Can you work these out from the model? Positions are in its coordinate system, mm. Face numbers are marked on the shaded views. A direction names the side the tool comes from. Coordinates: 2 decimals unless noted, no trailing zeros. Order: outer loops, then holes, each group sorted by start corner. A loop starts at its lowest first (then second) coordinate and runs counter-clockwise, first axis right, second up. Notation, with made-up numbers: (-29, -25.5) -> (-10, -25.5) arc R9 ccw to (-10, -13.5) -> close; hole circle Ø4 at (1, 87). An arc over 180 degrees is marked (long way). Write item = value, one per line.
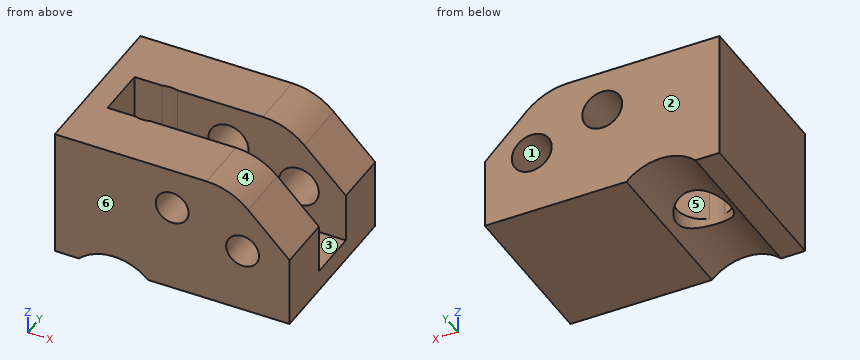
```python
from build123d import *

# Parameters (mm, degrees)
CYLINDER060_R          = 2.3
CYLINDER060_DEPTH      = 62
CYLINDER062_R          = 4.2
CYLINDER062_DEPTH      = 24
CYLINDER062_ROLL_ANGLE = 90
BOX001024_W            = 23
BOX001024_H            = 4.4
BOX001024_DEPTH        = 13
CYLINDER056_R          = 1.7
CYLINDER056_DEPTH      = 20
CYLINDER056_ROLL_ANGLE = 90
CYLINDER057_R          = 1.7
CYLINDER057_DEPTH      = 20
CYLINDER057_ROLL_ANGLE = 90
CYLINDER059_R          = 1.4
CYLINDER059_DEPTH      = 20
CYLINDER059_ROLL_ANGLE = 90
CYLINDER058_R          = 1.4
CYLINDER058_DEPTH      = 20
CYLINDER058_ROLL_ANGLE = 90
BOX001025_W            = 10
BOX001025_H            = 27
BOX001025_DEPTH        = 10
BOX001022_W            = 23
BOX001022_H            = 14
BOX001022_DEPTH        = 11
CHAMFER003_SIZE        = 8
FILLET007_R            = 5


with BuildPart() as cylinder060:
    # Cylinder060 → Cylinder060 (new body)
    with BuildSketch(Plane.XY.offset(-56)):
        Circle(CYLINDER060_R)
    extrude(amount=CYLINDER060_DEPTH)


with BuildPart() as cylinder062:
    # Cylinder062 → Cylinder062 (new body)
    with BuildSketch(Plane.XY):
        Circle(CYLINDER062_R)
    extrude(amount=CYLINDER062_DEPTH)


with BuildPart() as cylinder062_1:
    # Cylinder062 roll: moved
    add(cylinder062.part.rotate(Axis((0, 0, 0), (1, 0, 0)), CYLINDER062_ROLL_ANGLE))


with BuildPart() as cylinder062_2:
    # Cylinder062 placement: moved
    add(cylinder062_1.part.moved(Location((0, 11, -52))))


with BuildPart() as cube022:
    # Box001024 → Box001024 (new body)
    with BuildSketch(Plane(origin=(-3, -2.2, -47.2), x_dir=(1, 0, 0), z_dir=(0, 0, 1))):
        with Locations((11.5, 2.2)):
            Rectangle(BOX001024_W, BOX001024_H)
    extrude(amount=BOX001024_DEPTH)


with BuildPart() as cylinder056:
    # Cylinder056 → Cylinder056 (new body)
    with BuildSketch(Plane.XY):
        Circle(CYLINDER056_R)
    extrude(amount=CYLINDER056_DEPTH)


with BuildPart() as cylinder056_1:
    # Cylinder056 roll: moved
    add(cylinder056.part.rotate(Axis((0, 0, 0), (1, 0, 0)), CYLINDER056_ROLL_ANGLE))


with BuildPart() as cylinder056_2:
    # Cylinder056 placement: moved
    add(cylinder056_1.part.moved(Location((11, 19, -43.5))))


with BuildPart() as cylinder057:
    # Cylinder057 → Cylinder057 (new body)
    with BuildSketch(Plane.XY):
        Circle(CYLINDER057_R)
    extrude(amount=CYLINDER057_DEPTH)


with BuildPart() as cylinder057_1:
    # Cylinder057 roll: moved
    add(cylinder057.part.rotate(Axis((0, 0, 0), (1, 0, 0)), CYLINDER057_ROLL_ANGLE))


with BuildPart() as cylinder057_2:
    # Cylinder057 placement: moved
    add(cylinder057_1.part.moved(Location((5, 19, -41.5))))


with BuildPart() as cylinder059:
    # Cylinder059 → Cylinder059 (new body)
    with BuildSketch(Plane.XY):
        Circle(CYLINDER059_R)
    extrude(amount=CYLINDER059_DEPTH)


with BuildPart() as cylinder059_1:
    # Cylinder059 roll: moved
    add(cylinder059.part.rotate(Axis((0, 0, 0), (1, 0, 0)), CYLINDER059_ROLL_ANGLE))


with BuildPart() as cylinder059_2:
    # Cylinder059 placement: moved
    add(cylinder059_1.part.moved(Location((5, -1, -41.5))))


with BuildPart() as fusion074:
    # Cylinder058 → Cylinder058 (new body)
    with BuildSketch(Plane.XY):
        Circle(CYLINDER058_R)
    extrude(amount=CYLINDER058_DEPTH)


with BuildPart() as fusion074_1:
    # Cylinder058 roll: moved
    add(fusion074.part.rotate(Axis((0, 0, 0), (1, 0, 0)), CYLINDER058_ROLL_ANGLE))


with BuildPart() as fusion074_2:
    # Cylinder058 placement: moved
    add(fusion074_1.part.moved(Location((11, -1, -43.5))))

    # Fusion074: union Cylinder056, Cylinder057, Cylinder059
    add(cylinder056_2.part)
    add(cylinder057_2.part)
    add(cylinder059_2.part)


with BuildPart() as cube023:
    # Box001025 → Box001025 (new body)
    with BuildSketch(Plane(origin=(15, -13, -44), x_dir=(1, 0, 0), z_dir=(0, 0, 1))):
        with Locations((5, 13.5)):
            Rectangle(BOX001025_W, BOX001025_H)
    extrude(amount=BOX001025_DEPTH)


with BuildPart() as cut_lever_block:
    # Box001022 → Box001022 (new body)
    with BuildSketch(Plane(origin=(-5, -7, -42), x_dir=(1, 0, 0), z_dir=(0, 0, 1))):
        with Locations((11.5, 7)):
            Rectangle(BOX001022_W, BOX001022_H)
    extrude(amount=BOX001022_DEPTH)

    # Chamfer003
    chamfer003_edges = [cut_lever_block.edges().sort_by_distance(p)[0] for p in [
        (18, 0, -31),
    ]]
    chamfer(chamfer003_edges, length=CHAMFER003_SIZE)

    # Fillet007
    fillet007_edges = [cut_lever_block.edges().sort_by_distance(p)[0] for p in [
        (10, 0, -31),
    ]]
    fillet(fillet007_edges, radius=FILLET007_R)

    # Cut022: cut Cube023
    add(cube023.part, mode=Mode.SUBTRACT)


with BuildPart() as cut_lever_block_1:
    # Cut022 placement: moved
    add(cut_lever_block.part.moved(Location((0, 0, -7))))

    # Cut027: cut Fusion074
    add(fusion074_2.part, mode=Mode.SUBTRACT)

    # Cut028: cut Cube022
    add(cube022.part, mode=Mode.SUBTRACT)

    # Cut029: cut Cylinder062
    add(cylinder062_2.part, mode=Mode.SUBTRACT)

    # Cut030: cut Cylinder060
    add(cylinder060.part, mode=Mode.SUBTRACT)


with BuildPart() as cut_lever_block_2:
    # Cut030 placement: moved
    add(cut_lever_block_1.part.moved(Location((0, 0, -6))))


solid = cut_lever_block_2.part
```
Item 1: I'm going to push flat-ended pins straight in: P1, Ø1.3, axis at x = 11.5, y = 0, coming from the +Z side; P2, Ø2, axis at y = -0.5, z = -46.5, coming from the +X side. Where does each tip first touch, or does it pass through?
A:
P1 = -53.2
P2 = -3
Item 2: I want a section at D-D, the plane x = 5. Please give me the cut outline in (y, z).
A:
outline = (-7, -55) -> (7, -55) -> (7, -49.2) -> (2.2, -49.2) -> (2.2, -53.2) -> (-2.2, -53.2) -> (-2.2, -48.9) -> (-7, -48.9) -> close; (-7, -46.1) -> (-2.2, -46.1) -> (-2.2, -44) -> (-7, -44) -> close; (2.2, -45.8) -> (7, -45.8) -> (7, -44) -> (2.2, -44) -> close
Item 3: If we mould it in two halves opening along Y, with no side actions, what happens to the marked faces 4, 5 and 6? For each: pulls with the +Y half, pulls with the -Y half, needs draft (parallel to the pull), parting line crosses it, or undercut.
A:
face_4 = needs draft
face_5 = undercut
face_6 = pulls with the -Y half
Item 4: I want a section at B-B, the plane z = -49.5. Please give me the cut outline in (x, y), plus the area to 3 significant figures.
A:
outline = (-5, -7) -> (9.6, -7) -> (9.6, -2.2) -> (0.67, -2.2) arc R2.3 cw to (-0.67, -2.2) -> (-3, -2.2) -> (-3, 2.2) -> (-0.67, 2.2) arc R2.3 cw to (0.67, 2.2) -> (9.3, 2.2) -> (9.3, 7) -> (-5, 7) -> close; (12.4, -7) -> (15, -7) -> (15, -2.2) -> (12.4, -2.2) -> close; (12.7, 2.2) -> (15, 2.2) -> (15, 7) -> (12.7, 7) -> close
area = 171 mm2
Item 5: If I drill on probe 1 along Y at (x, z) = (8.5, -51); probe 2 along X at (y, z) = (-4.35, -49.5); probe 3 along Z at (x, y) = (5, -4.6), over which ranges is the centre line in solid material (lowest first)?
A:
probe_1 = -7 to -2.2, 2.2 to 7
probe_2 = -5 to 9.6, 12.4 to 15
probe_3 = -55 to -48.9, -46.1 to -44
Item 6: For the marked faces 1, 2 and 3, which set-ups out of +Z, -Z, +X, -X, +Y, -Y let a thin tool reach every point of the face, with its end or its side?
A:
face_1 = +Y
face_2 = +Z, -Z, +X, -X, +Y
face_3 = +Z, +X
Item 7: I want a section at C-C, the plane y = 4.5. Please give me the cut outline in (x, z).
A:
outline = (-5, -55) -> (-2.94, -55) arc R4.2 cw to (2.94, -55) -> (15, -55) -> (15, -49) -> (11.46, -45.46) arc R5 ccw to (7.93, -44) -> (-5, -44) -> close; hole circle Ø3.4 at (5, -47.5); hole circle Ø3.4 at (11, -49.5)
Item 8: I want a section at A-A, the plane x = 0. Please give me the cut outline in (y, z), plus the area to 3 significant figures.
A:
outline = (-7, -53.8) -> (-2.3, -53.8) -> (-2.3, -44) -> (-7, -44) -> close; (2.3, -53.8) -> (7, -53.8) -> (7, -44) -> (2.3, -44) -> close
area = 92.1 mm2
